Autodesk Inventor part; units mm, degrees
ref_plane "C1_XY" through (0, 0, 0) normal (0, 0, 1) x (1, 0, 0)
ref_plane "C1_YZ" through (0, 0, 0) normal (1, 0, 0) x (0, 1, 0)
ref_plane "C1_ZX" through (0, 0, 0) normal (0, 1, 0) x (0, 0, 1)
sketch "Sketch_1" plane through (0, 0, 0) normal (0, 0, 1) x (1, 0, 0)
  line L0 (-15, -4) -> (-15, -13)
  arc A0 (-15, -13) -> (-13, -15) centre (-13, -13) ccw
  line L1 (-13, -15) -> (-4, -15)
  line L2 (-4, -15) -> (-4, -13)
  line L3 (-4, -13) -> (-8.25, -13)
  line L4 (-8.25, -13) -> (-8.25, -9.6642)
  line L5 (-8.25, -9.6642) -> (-4.5858, -6)
  line L6 (-4.5858, -6) -> (-0.5196, -6)
  line L7 (-0.5196, -6) -> (0, -5.7)
  line L8 (0, -5.7) -> (0.5196, -6)
  line L9 (0.5196, -6) -> (4.5858, -6)
  line L10 (4.5858, -6) -> (8.25, -9.6642)
  line L11 (8.25, -9.6642) -> (8.25, -13)
  line L12 (8.25, -13) -> (4, -13)
  line L13 (4, -13) -> (4, -15)
  line L14 (4, -15) -> (13, -15)
  arc A1 (13, -15) -> (15, -13) centre (13, -13) ccw
  line L15 (15, -13) -> (15, -4)
  line L16 (15, -4) -> (13, -4)
  line L17 (13, -4) -> (13, -8.25)
  line L18 (13, -8.25) -> (9.6642, -8.25)
  line L19 (9.6642, -8.25) -> (6, -4.5858)
  line L20 (6, -4.5858) -> (6, -0.5196)
  line L21 (6, -0.5196) -> (5.7, 0)
  line L22 (5.7, 0) -> (6, 0.5196)
  line L23 (6, 0.5196) -> (6, 4.5858)
  line L24 (6, 4.5858) -> (9.6642, 8.25)
  line L25 (9.6642, 8.25) -> (13, 8.25)
  line L26 (13, 8.25) -> (13, 4)
  line L27 (13, 4) -> (15, 4)
  line L28 (15, 4) -> (15, 13)
  arc A2 (15, 13) -> (13, 15) centre (13, 13) ccw
  line L29 (13, 15) -> (4, 15)
  line L30 (4, 15) -> (4, 13)
  line L31 (4, 13) -> (8.25, 13)
  line L32 (8.25, 13) -> (8.25, 9.6642)
  line L33 (8.25, 9.6642) -> (4.5858, 6)
  line L34 (4.5858, 6) -> (0.5196, 6)
  line L35 (0.5196, 6) -> (0, 5.7)
  line L36 (0, 5.7) -> (-0.5196, 6)
  line L37 (-0.5196, 6) -> (-4.5858, 6)
  line L38 (-4.5858, 6) -> (-8.25, 9.6642)
  line L39 (-8.25, 9.6642) -> (-8.25, 13)
  line L40 (-8.25, 13) -> (-4, 13)
  line L41 (-4, 13) -> (-4, 15)
  line L42 (-4, 15) -> (-13, 15)
  arc A3 (-13, 15) -> (-15, 13) centre (-13, 13) ccw
  line L43 (-15, 13) -> (-15, 4)
  line L44 (-15, 4) -> (-13, 4)
  line L45 (-13, 4) -> (-13, 8.25)
  line L46 (-13, 8.25) -> (-9.6642, 8.25)
  line L47 (-9.6642, 8.25) -> (-6, 4.5858)
  line L48 (-6, 4.5858) -> (-6, 0.5196)
  line L49 (-6, 0.5196) -> (-5.7, 0)
  line L50 (-5.7, 0) -> (-6, -0.5196)
  line L51 (-6, -0.5196) -> (-6, -4.5858)
  line L52 (-6, -4.5858) -> (-9.6642, -8.25)
  line L53 (-9.6642, -8.25) -> (-13, -8.25)
  line L54 (-13, -8.25) -> (-13, -4)
  line L55 (-13, -4) -> (-15, -4)
extrude "Extrusion1" add sketch "Sketch_1" against normal blind 223
sketch "Sketch2" plane through (0, 0, -223) normal (0, 0, -1) x (-1, 0, 0)
  point P0 (0, 0)
hole "Hole1" at (0, 0, -223) direction (0, 0, 1) diameter 6.8 depth 223
sketch "Sketch3" plane through (0, 0, -223) normal (0, 0, -1) x (-1, 0, 0)
  point P0 (-11.6, 11.6)
hole "Hole2" at (11.6, 11.6, -223) direction (0, 0, 1) diameter 4.2 depth 223
pattern_linear "Rectangular Pattern1" count 2 spacing 23.2 along (-1, 0, 0) count 2 spacing 23.2 along (0, -1, 0) of "Hole2"
ref_plane "C1_XY" through (0, 0, 0) normal (0, 0, 1) x (1, 0, 0)
ref_plane "C1_YZ" through (0, 0, 0) normal (1, 0, 0) x (0, 1, 0)
ref_plane "C1_ZX" through (0, 0, 0) normal (0, 1, 0) x (0, 0, 1)
ref_plane "to_frame_cap1_XY" through (0, 0, 0) normal (0, 0, 1) x (1, 0, 0)
ref_plane "to_frame_cap1_YZ" through (0, 0, 0) normal (1, 0, 0) x (0, 1, 0)
ref_plane "to_frame_cap1_ZX" through (0, 0, 0) normal (0, 1, 0) x (0, 0, 1)
ref_plane "to_frame_cap2_XY" through (0, 0, -223) normal (0, 0, -1) x (1, 0, 0)
ref_plane "to_frame_cap2_YZ" through (0, 0, -223) normal (1, 0, 0) x (0, -1, 0)
ref_plane "to_frame_cap2_ZX" through (0, 0, -223) normal (0, -1, 0) x (0, 0, -1)
properties part number "HFS6-3030-223"
The model under review builds one solid part; all positions refer to its coordinate system, in mm. A direction names the side the tool comes from. Coordinates: 2 decimals unless noted, no trailing zeros. Write item = value, one per line.
(1) For P1, Ø1.2, axis at y = -2.5, z = -69.5, coming from the +X side; P2, Ø0.6, axis at y = -14.5, z = -86, coming from the +X side; P3, Ø4, axis at x = 11.6, y = 11.6, coming from the -Z side; P4, Ø1.6, axis at x = 14.5, z = -155.5, coming from the -Y side, all flat-tipped, find the tip position at first contact; note any pin that passes through.
Result sheet:
P1 = 6
P2 = 14.6
P3 = through
P4 = -14.87
(2) Machinability: for faces 4 (the face through (-6, -13, -110)), 5 (the face through (8, -15, -110)), which of the approach directions +Z, -Z, +X, -X, +Y, -Y give a long, thin tool a straight path to every point of the face, cutting with its end or side? Answer none if there is none.
Result sheet:
face_4 = +Z, -Z
face_5 = +Z, -Z, +X, -X, -Y
(3) Consider section A-A, the plane z = -138. State how many separate pieces and enclosed holes the cut face has, then the cut area to 3 significant figures.
Result sheet:
separate_pieces = 1
enclosed_holes = 5
area = 332 mm^2
(4) For line 1 (X direction, y = -11.6, z = -130.5); line 2 (Y direction, x = -11.25, z = -101); line 3 (Y direction, x = 12.25, z = -35), list the stretches that pass through material, from the lowest coordinate up. Write a range as [from, to].
Result sheet:
line_1 = [-15, -13.7], [-9.5, -8.25], [8.25, 9.5], [13.7, 15]
line_2 = [-15, -13.67], [-9.53, -8.25], [8.25, 9.53], [13.67, 15]
line_3 = [-15, -13.6], [-9.6, -8.25], [8.25, 9.6], [13.6, 15]
(5) Mouldability with a two-part tool opening along X and no side actions: class faces 1 (the face through (3, -6, -110)), 2 (the face through (-4, 0, 0)), 3 (the face through (-15, -8, -110)) as pulls with the +X half, pulls with the -X half, needs draft (parallel to the pull), parting line crosses it, or undercut.
Result sheet:
face_1 = undercut
face_2 = needs draft
face_3 = pulls with the -X half
